```python
from build123d import *

# Parameters (mm, degrees)
F3_R     = 4.7625
F3_R_2   = 31.75
F3_R_3   = 25.4
F8_DEPTH = 9.525


with BuildPart() as f8:
    # F3 (on offset) → F8 (new body)
    with BuildSketch(Plane.YZ.offset(-203.2)):
        with BuildLine():
            ThreePointArc((504.085483, 127.539883), (500.512376, 128.192005), (497.881204, 130.69586))
            ThreePointArc((497.881204, 130.69586), (467.968772, 149.729662), (435.329623, 135.883177))
            ThreePointArc((435.329623, 135.883177), (428.605586, 130.10633), (420.305835, 126.992045))
            ThreePointArc((420.305835, 126.992045), (418.631702, 126.906277), (416.99346, 127.261584))
            ThreePointArc((416.99346, 127.261584), (410.909202, 128.18666), (404.930309, 126.728302))
            ThreePointArc((404.930309, 126.728302), (403.577562, 126.277317), (402.15829, 126.139551))
            ThreePointArc((402.15829, 126.139551), (391.400337, 128.718459), (382.759018, 135.62584))
            ThreePointArc((382.759018, 135.62584), (351.898546, 149.842293), (321.961786, 133.771613))
            ThreePointArc((321.961786, 133.771613), (318.79924, 131.420238), (314.858479, 131.387525))
            ThreePointArc((314.858479, 131.387525), (304.601343, 131.163607), (296.623197, 124.713168))
            ThreePointArc((296.623197, 124.713168), (293.400016, 122.121405), (289.264455, 122.064311))
            ThreePointArc((289.264455, 122.064311), (286.078264, 122.760136), (282.817118, 122.790184))
            ThreePointArc((282.817118, 122.790184), (278.969036, 123.659479), (276.37693, 126.633432))
            ThreePointArc((276.37693, 126.633432), (246.538925, 149.498093), (211.600982, 135.62584))
            ThreePointArc((211.600982, 135.62584), (203.667081, 129.078189), (193.787021, 126.214112))
            ThreePointArc((193.787021, 126.214112), (192.392802, 126.258483), (191.041911, 126.606203))
            ThreePointArc((191.041911, 126.606203), (185.42, 127.635), (179.798089, 126.606203))
            ThreePointArc((179.798089, 126.606203), (178.447198, 126.258483), (177.052979, 126.214112))
            ThreePointArc((177.052979, 126.214112), (167.172919, 129.078189), (159.239018, 135.62584))
            ThreePointArc((159.239018, 135.62584), (126.556336, 149.742993), (96.478796, 130.69586))
            ThreePointArc((96.478796, 130.69586), (93.847624, 128.192005), (90.274517, 127.539883))
            ThreePointArc((90.274517, 127.539883), (72.66432, 111.76), (90.274517, 95.980117))
            ThreePointArc((90.274517, 95.980117), (93.847624, 95.327995), (96.478796, 92.82414))
            ThreePointArc((96.478796, 92.82414), (126.556336, 73.777007), (159.239018, 87.89416))
            ThreePointArc((159.239018, 87.89416), (167.172919, 94.441811), (177.052979, 97.305888))
            ThreePointArc((177.052979, 97.305888), (178.447198, 97.261517), (179.798089, 96.913797))
            ThreePointArc((179.798089, 96.913797), (185.42, 95.885), (191.041911, 96.913797))
            ThreePointArc((191.041911, 96.913797), (192.392802, 97.261517), (193.787021, 97.305888))
            ThreePointArc((193.787021, 97.305888), (203.667081, 94.441811), (211.600982, 87.89416))
            ThreePointArc((211.600982, 87.89416), (242.341876, 73.674248), (272.259375, 89.553535))
            ThreePointArc((272.259375, 89.553535), (275.440775, 91.886366), (279.385822, 91.890269))
            ThreePointArc((279.385822, 91.890269), (289.701554, 92.056216), (297.736803, 98.527432))
            ThreePointArc((297.736803, 98.527432), (300.959984, 101.119195), (305.095545, 101.176289))
            ThreePointArc((305.095545, 101.176289), (308.322678, 100.475909), (311.62489, 100.458336))
            ThreePointArc((311.62489, 100.458336), (315.473668, 99.611242), (318.081479, 96.656587))
            ThreePointArc((318.081479, 96.656587), (348.184283, 73.973264), (383.059023, 88.272373))
            ThreePointArc((383.059023, 88.272373), (392.162049, 95.558021), (403.56111, 98.008978))
            ThreePointArc((403.56111, 98.008978), (404.685964, 97.885867), (405.771107, 97.565059))
            ThreePointArc((405.771107, 97.565059), (411.310239, 96.454986), (416.887372, 97.3549))
            ThreePointArc((416.887372, 97.3549), (418.651149, 97.706509), (420.442765, 97.549504))
            ThreePointArc((420.442765, 97.549504), (428.371848, 94.199323), (434.726695, 88.393293))
            ThreePointArc((434.726695, 88.393293), (467.486497, 73.753424), (497.881204, 92.82414))
            ThreePointArc((497.881204, 92.82414), (500.512376, 95.327995), (504.085483, 95.980117))
            ThreePointArc((504.085483, 95.980117), (521.69568, 111.76), (504.085483, 127.539883))
        make_face()
        with Locations((88.53932, 111.76)):
            Circle(F3_R, mode=Mode.SUBTRACT)
        with Locations((129.54, 111.76)):
            Circle(F3_R_2, mode=Mode.SUBTRACT)
        with Locations((185.42, 111.76)):
            Circle(F3_R, mode=Mode.SUBTRACT)
        with Locations((284.3022, 106.9848)):
            Circle(F3_R, mode=Mode.SUBTRACT)
        with Locations((241.3, 111.76)):
            Circle(F3_R_2, mode=Mode.SUBTRACT)
        with Locations((353.06, 111.76)):
            Circle(F3_R_2, mode=Mode.SUBTRACT)
        with Locations((464.82, 111.76)):
            Circle(F3_R_2, mode=Mode.SUBTRACT)
        with Locations((505.82068, 111.76)):
            Circle(F3_R, mode=Mode.SUBTRACT)
        with Locations((310.0578, 116.2558)):
            Circle(F3_R, mode=Mode.SUBTRACT)
        with Locations((411.610311, 112.327149)):
            Circle(F3_R, mode=Mode.SUBTRACT)
        with Locations((129.54, 111.76)):
            Circle(F3_R_2)
        with Locations((129.54, 111.76)):
            Circle(F3_R_3, mode=Mode.SUBTRACT)
        with Locations((241.3, 111.76)):
            Circle(F3_R_2)
        with Locations((241.3, 111.76)):
            Circle(F3_R_3, mode=Mode.SUBTRACT)
        with Locations((353.06, 111.76)):
            Circle(F3_R_2)
        with Locations((353.06, 111.76)):
            Circle(F3_R_3, mode=Mode.SUBTRACT)
        with Locations((464.82, 111.76)):
            Circle(F3_R_2)
        with Locations((464.82, 111.76)):
            Circle(F3_R_3, mode=Mode.SUBTRACT)
    extrude(amount=F8_DEPTH)


solid = f8.part
```
Design review of the part built by this model. Coordinates are the model's own, in mm. A direction names the side the tool comes from. Coordinates: 2 decimals unless noted, no trailing zeros. Loops run counter-clockwise (first coordinate to the right, second up) from the corner with the lowest first, then second, coordinate; pieces in that order, holes last. Notation, with made-up numbers: (-16, 80) -> (28, 80) arc R36 cw to (28, 115) -> close; hole circle Ø8 at (49.5, 4). An arc over 180 degrees is marked (long way). Answer as a JSON object with one key per item and string values.
Q1. Take a section at A-A on y = 185.42. Give the boundary of the cut face in (x, z) (1 decimal).
Answer block:
{"outline": "(-203.2, 95.9) -> (-193.7, 95.9) -> (-193.7, 107) -> (-203.2, 107) -> close; (-203.2, 116.5) -> (-193.7, 116.5) -> (-193.7, 127.6) -> (-203.2, 127.6) -> close"}
Q2. The part is to be moulded in two halves that separate along Z. For faces 1 (the cylindrical face through (-198.504, 293.455, 122.142)), 2 (the cylindrical face through (-198.504, 264.763, 102.032)), 3 (the cylindrical face through (-198.504, 289.563, 92.007)), say which applies: +Z half, -Z half, draft (parallel to the pull), parting line (faces both ways), or undercut.
Answer block:
{"face 1": "+Z half", "face 2": "undercut", "face 3": "-Z half"}
Q3. Take a section at C-C on x = -197.5. Give the number of separate pieces and of enclosed holes in the cut face, plus the area to 3 significant figures.
Answer block:
{"separate pieces": "1", "enclosed holes": "10", "area": "14,300 mm^2"}
Q4. Take a section at B-B on y = 129.54. Give the boundary of the cut face in (x, z) (3 decimals), plus the area to 3 significant figures.
Answer block:
{"outline": "(-203.2, 73.66) -> (-193.675, 73.66) -> (-193.675, 86.36) -> (-203.2, 86.36) -> close; (-203.2, 137.16) -> (-193.675, 137.16) -> (-193.675, 149.86) -> (-203.2, 149.86) -> close", "area": "242 mm^2"}
Q5. To check wall thickness, follow L1, parallel to Y at x = -202.25, z = 125; L2, parallel to Z at x = -198, y = 129; L3, parallel to Y at x = -200.5, z = 85. State the ranges of each line that lie inside material, in increasing order.
Answer block:
{"L1": "y = 79.78 to 107.86, 151.22 to 219.62, 262.98 to 277.38, 296.81 to 331.38, 374.74 to 443.14, 486.5 to 514.58", "L2": "z = 73.66 to 86.37, 137.15 to 149.86", "L3": "y = 102.42 to 156.66, 214.18 to 268.42, 325.94 to 380.18, 437.7 to 491.94"}
Q6. Tool access review of faces 4 (the cylindrical face through (-198.5, 167.3, 129.01)), 5 (the cylindrical face through (-198.504, 87.919, 116.482)), 6 (the cylindrical face through (-198.5, 203.54, 94.51)): name each direction out of +Z, -Z, +X, -X, +Y, -Y from which nothing blocks a thin tool from reaching the whole face with its end or side.
Answer block:
{"face 4": "+Z, +X, -X", "face 5": "+X, -X", "face 6": "-Z, +X, -X"}
